```python
from build123d import *

# Parameters (mm, degrees)
F0_W     = 42
F0_H     = 24.59859317
F0_R     = 1.25
F1_DEPTH = 5
F3_DEPTH = 42
F5_R     = 1.25
F6_DEPTH = 16


with BuildPart() as f1:
    # F0 (on Top) → F1 (new body)
    with BuildSketch(Plane.XY):
        with Locations((21, 12.299296585)):
            Rectangle(F0_W, F0_H)
        with Locations((3.5, 22.09859317)):
            Circle(F0_R, mode=Mode.SUBTRACT)
        with Locations((38.5, 22.09859317)):
            Circle(F0_R, mode=Mode.SUBTRACT)
    extrude(amount=F1_DEPTH)

    # F2 (on face) → F3 (join, through all)
    with BuildSketch(Plane(origin=(0, 0, 0), x_dir=(0, -1, 0), z_dir=(-1, 0, 0))):
        Polygon((0, 5), (0, 0), (3, 0), (3, 12), (0, 12), (-5, 10), (0, 8), align=None)
    extrude(amount=-F3_DEPTH)

    # F5 (on Right) → F6 (join)
    with BuildSketch(Plane.YZ):
        Polygon((3.5, -19), (3.5, 0), (-3, 0), (1.4603033196, -35), (35.5, -35), (35.5, -19), (30.75, -19), (30.75, -31), (8.25, -31), (8.25, -19), align=None)
        with Locations((5.5, -25)):
            Circle(F5_R, mode=Mode.SUBTRACT)
        with Locations((33.5, -25)):
            Circle(F5_R, mode=Mode.SUBTRACT)
    extrude(amount=F6_DEPTH)


solid = f1.part
```
Design review of the part built by this model. Coordinates are the model's own, in mm. A direction names the side the tool comes from. Round coordinates to 2 decimals unless told otherwise and drop trailing zeros. Order: outer loops, then holes, each group sorted by start corner. A loop starts at its lowest first (then second) coordinate and runs counter-clockwise, first axis right, second up. Notation, with made-up numbers: (0, 31) - (16, 31) arc R15 cw to (16, 60) - close; hole circle Ø1 at (43.5, -4). An arc over 180 degrees is marked (long way). One line per question, with ' | ' between items.
Item 1: Draft analysis for pull direction Y (two halves, no side actions). For faces 4 (the face through (8, 8.25, -25)), 5 (the face through (8, 35.5, -27)), 6 (the face through (21, -2, 12)), state which applies: +Y half, -Y half, draft (parallel to the pull), parting line (faces both ways), or undercut.
Checks:
face 4: undercut | face 5: +Y half | face 6: draft
Item 2: For P1, Ø1.4, axis at x = 10, y = 33.5, coming from the +Z side; P2, Ø5, axis at x = 10, z = -6.5, coming from the -Y side; P3, Ø7.5, axis at x = 18, y = 15, coming from the +Z side; P4, Ø17.5, axis at x = 12, z = -12, coming from the +Y side, all flat-tipped, find the tip position at first contact; note any pin that passes through.
Checks:
P1: z = -19 | P2: y = -2.49 | P3: z = 5 | P4: y = 35.5
Item 3: Take a section at D-D, the plane z = -25. Write out the cut boundary in (x, y), then the cut area to 3 significant figures.
Checks:
outline: (0, 0.19) - (16, 0.19) - (16, 4.25) - (0, 4.25) - close; (0, 6.75) - (16, 6.75) - (16, 8.25) - (0, 8.25) - close; (0, 30.75) - (16, 30.75) - (16, 32.25) - (0, 32.25) - close; (0, 34.75) - (16, 34.75) - (16, 35.5) - (0, 35.5) - close | area: 125 mm²
Item 4: Take a section at A-A, the plane y = 11.5. Write out the cut boundary in (x, z).
Checks:
outline: (0, -35) - (16, -35) - (16, -31) - (0, -31) - close; (0, 0) - (42, 0) - (42, 5) - (0, 5) - close
Item 5: Take a section at C-C, the plane x = 38.5. Write out the cut boundary in (y, z), then the cut area to 3 significant figures.
Checks:
outline: (-3, 0) - (20.85, 0) - (20.85, 5) - (0, 5) - (0, 8) - (5, 10) - (0, 12) - (-3, 12) - close; (23.35, 0) - (24.6, 0) - (24.6, 5) - (23.35, 5) - close | area: 156 mm²
Item 6: Wall thickness on line 1 (Z direction, x = 8.5, y = 33.5); line 2 (Z direction, x = 10.5, y = 6.5); line 3 (Y direction, x = 38.5, z = 3.7): over which ranges is each line inside the solid? List them lowest first. Write a range as [from, to].
Checks:
line 1: [-35, -26.25], [-23.75, -19] | line 2: [-35, -25.75], [-24.25, -19], [0, 5] | line 3: [-3, 20.85], [23.35, 24.6]
Item 7: Machinability: for faces 1 (the face through (21, 11, 0)), 2 (the face through (8, 20, -31)), 3 (the face through (21, 0, 7)), which of the approach directions +Z, -Z, +X, -X, +Y, -Y give a long, thin tool a straight path to every point of the face, cutting with its end or side? Answer none if there is none.
Checks:
face 1: +X, +Y | face 2: +X, -X | face 3: +X, -X, +Y
Item 8: Take a section at B-B, the plane x = 3.5. Write out the cut boundary in (y, z).
Checks:
outline: (-3, 0) - (1.46, -35) - (35.5, -35) - (35.5, -19) - (30.75, -19) - (30.75, -31) - (8.25, -31) - (8.25, -19) - (3.5, -19) - (3.5, 0) - (20.85, 0) - (20.85, 5) - (0, 5) - (0, 8) - (5, 10) - (0, 12) - (-3, 12) - close; (23.35, 0) - (24.6, 0) - (24.6, 5) - (23.35, 5) - close; hole circle Ø2.5 at (5.5, -25); hole circle Ø2.5 at (33.5, -25)
